Autodesk Inventor part; units mm, degrees
ref_plane "YZ Plane" through (0, 0, 0) normal (1, 0, 0) x (0, 1, 0)
ref_plane "XZ Plane" through (0, 0, 0) normal (0, 1, 0) x (-1, 0, 0)
ref_plane "XY Plane" through (0, 0, 0) normal (0, 0, 1) x (1, 0, 0)
sketch "Sketch1" plane through (0, 0, 0) normal (0, 1, 0) x (-1, 0, 0)
  circle A0 centre (0, 0) radius 32.5
  circle A1 centre (0, 0) radius 35.5
  dimension "d0" = 65
  dimension "d1" = 71
extrude "Extrusion1" add sketch "Sketch1" along normal blind 8
extrude "Extrusion2" add sketch "Sketch1" along normal blind 3 contours A0
fillet "Fillet1" radius 2 2 edges at (35.5, 0, 0) (32.5, 3, 0)
fillet "Fillet2" radius 1.5 2 edges at (32.5, 8, 0) (35.5, 8, 0)
sketch "Sketch2" plane through (0, 3, 0) normal (0, 1, 0) x (1, 0, 0)
  circle A0 centre (0, 0) radius 0.25
  circle A1 centre (0, 0) radius 2.5
  circle A2 centre (0, 2) radius 0.5
  line L0 (-0.5, 2) -> (-0.5, 1.5) construction
  line L1 (-0.5, 1.5) -> (-0.25, 0.892563) construction
  line L2 (-0.25, 0.892563) -> (0, 0.421283) construction
  spline S0 degree 3 poles (-0.5, 2) (-0.5, 1.5) (-0.25, 0.892563) (0, 0.421283) knots 1 1 1 1 2 2 2 2
  line L3 (-0.5, 1.5) -> (0.5, 1.5)
  line L4 (-0.25, 0.892563) -> (0.25, 0.892563)
  line L5 (0.5, 2) -> (0.5, 1.5) construction
  line L6 (0.5, 1.5) -> (0.25, 0.892563) construction
  line L7 (0.25, 0.892563) -> (0, 0.421283) construction
  spline S1 degree 3 poles (0.5, 2) (0.5, 1.5) (0.25, 0.892563) (0, 0.421283) knots 1 1 1 1 2 2 2 2
  dimension "d12" = 0.5
  dimension "d13" = 5
sketch "Sketch2 outline for Extrusion4" plane through (0, 3, 0) normal (0, 1, 0) x (1, 0, 0)
  circle A0 centre (0, 0) radius 0.25
  spline S0 degree 3 poles (0.5, 2) (0.5, 1.5) (0.25, 0.892563) (0, 0.421283) knots 0 0 0 0 1 1 1 1
  spline S1 degree 3 poles (-0.5, 2) (-0.5, 1.5) (-0.25, 0.892563) (0, 0.421283) knots 0 0 0 0 1 1 1 1
  arc A1 (0.5, 2) -> (-0.5, 2) centre (0, 2) ccw
extrude "Extrusion4" cut sketch "Sketch2 outline for Extrusion4" against normal blind 1
pattern_circular "Circular Pattern1" count 9 over 360 about axis through (0, -10, 0) along (0, 1, 0) of "Extrusion4"
properties part number "Orchid Coaster V4"
Geometry check sheet. Reference: the model listing, model coordinates, mm. Coordinates: 2 decimals unless noted, no trailing zeros. Answer as a JSON object with one key per item and string values. Group by question number.
Item 1: Scan lines: probe 1 along Z at (x, y) = (0, 5.5); probe 2 along Y at (x, z) = (12, -3); probe 3 along Z at (x, y) = (-22, 7.25). Record each from-to range of solid material in increasing order.
Item 2: Draft check along X on faces 1 (the face through (-1, 2, -1)), 2 (the face through (1, 2, -1)), 3 (the face through (0, 0, 0)), 4 (the face through (7.696, 4.219, 34.656)). Enter one of: +X half, -X half, draft (parallel to the pull), parting line (faces both ways), or undercut.
Item 3: Depth check by flat-ended pin: pin 1 Ø1.1 at (x, z) = (0, -1.5) entering from +Y; pin 2 Ø12 at (x, z) = (-13.5, 21.5) entering from +Y; pin 3 Ø0.6 at (x, z) = (1.5, 1) entering from +Y. Enter the tip coordinate at first touch or a pass-through.
Resolved:
{
 "1": {"probe 1": "-35.5 to -32.5, 32.5 to 35.5", "probe 2": "0 to 3", "probe 3": "-27.6 to -24.19, 24.19 to 27.6"},
 "2": {"face 1": "undercut", "face 2": "undercut", "face 3": "draft", "face 4": "parting line"},
 "3": {"pin 1": "y = 3", "pin 2": "y = 3.21", "pin 3": "y = 2"}
}
